Read the model definition and answer for the solid it produces. Units are mm, in the model's axes. A direction names the side the tool comes from. Give positions to 0.01 mm unless a question says otherwise; leave off trailing zeros. Loops run counter-clockwise (first coordinate to the right, second up) from the corner with the lowest first, then second, coordinate; pieces in that order, holes last. Notation, with made-up numbers: (75, 58.5) - (106, 58.5) arc R29 ccw to (106, 84.5) - close; hole circle Ø4 at (30.25, 24.5). An arc over 180 degrees is marked (long way). Write item = value, one per line.
```python
from build123d import *

# Parameters (mm, degrees)
SKETCH1_W           = 42
SKETCH1_H           = 40
SKETCH1_R           = 2
SKETCH1_R_2         = 4
BOSS_EXTRUDE1_DEPTH = 3
SKETCH2_W           = 3
SKETCH2_H           = 40
BOSS_EXTRUDE2_DEPTH = 38
SKETCH3_W           = 40
SKETCH3_H           = 3
BOSS_EXTRUDE3_DEPTH = 40
CUT_EXTRUDE3_DEPTH  = 3


with BuildPart() as part:
    # Sketch1 → Boss-Extrude1 (new body)
    with BuildSketch(Plane(origin=(0, 0, 0), x_dir=(1, 0, 0), z_dir=(0, 1, 0))):
        Rectangle(SKETCH1_W, SKETCH1_H)
        with Locations(Location((-16, 15, 0), (0, 0, 270))):
            Circle(SKETCH1_R, mode=Mode.SUBTRACT)
        with Locations(Location((-16, -15, 0), (0, 0, 270))):
            Circle(SKETCH1_R, mode=Mode.SUBTRACT)
        with Locations(Location((-11, 0, 0), (0, 0, 270))):
            Circle(SKETCH1_R_2, mode=Mode.SUBTRACT)
    extrude(amount=BOSS_EXTRUDE1_DEPTH)

    # Sketch2 → Boss-Extrude2 (add)
    with BuildSketch(Plane(origin=(0, 3, 0), x_dir=(1, 0, 0), z_dir=(0, 1, 0))):
        with Locations((19.5, 0)):
            Rectangle(SKETCH2_W, SKETCH2_H)
    extrude(amount=BOSS_EXTRUDE2_DEPTH)

    # Sketch3 → Boss-Extrude3 (add)
    with BuildSketch(Plane(origin=(21, 0, 0), x_dir=(0, 0, -1), z_dir=(1, 0, 0))):
        with Locations((0, 39.5)):
            Rectangle(SKETCH3_W, SKETCH3_H)
    extrude(amount=BOSS_EXTRUDE3_DEPTH)

    # Sketch8 → Cut-Extrude3 (cut)
    with BuildSketch(Plane.XZ.offset(-38)):
        Polygon((21, -20), (61, 20), (61, -20), align=None)
    extrude(amount=-CUT_EXTRUDE3_DEPTH, mode=Mode.SUBTRACT)


solid = part.part
```
1) The mould has two halves that part along Z. Classify faces 4 (the face through (-14, 1, -15)), 5 (the face through (20, 20, 20)), 6 (the face through (-2, 3, 0)): pulls with the +Z half, pulls with the -Z half, needs draft (parallel to the pull), parting line crosses it, or undercut.
Output:
face_4 = undercut
face_5 = pulls with the +Z half
face_6 = needs draft
2) Find the intervals of material crossed by probe 1 along X at (y, z) = (0.95, 15); probe 2 along X at (y, z) = (0.6, 0); probe 3 along X at (y, z) = (29.5, -5), in increasing order.
Output:
probe_1 = -21 to -18, -14 to 21
probe_2 = -21 to -15, -7 to 21
probe_3 = 18 to 21
3) A cutting plane is placed at D-D on x = 0. Determine the outline of the cut face in (y, z), then the cut area to 3 significant figures.
Output:
outline = (0, -20) - (3, -20) - (3, 20) - (0, 20) - close
area = 120 mm²
4) Each of these flat-tipped pins is pushed along its axis until it touches: P1, Ø10.5, axis at x = -11, z = 0, coming from the +Y side; P2, Ø2, axis at y = 6, z = -7, coming from the +X side; P3, Ø12, axis at x = 36.5, z = -6.5, coming from the -Y side. Where does it stop, or does it pass through?
Output:
P1 = 3
P2 = 21
P3 = 38
5) A cutting plane is placed at C-C on z = -8.5. Determine the outline of the cut face in (x, y).
Output:
outline = (-21, 0) - (21, 0) - (21, 38) - (32.5, 38) - (32.5, 41) - (18, 41) - (18, 3) - (-21, 3) - close
6) A tool of negligible diameter and unlimited length cuts with its end or side. For faces 1 (the face through (21, 19, 0)), 2 (the face through (-14.905, 1.479, -0.867)), 3 (the face through (18, 22, 0)), from which of +Z, -Z, +X, -X, +Y, -Y can it reach the whole face along a straight path? Write none if from no direction.
Output:
face_1 = +Z, -Z, +X, -Y
face_2 = +Y, -Y
face_3 = +Z, -Z, -X, +Y
7) A cutting plane is placed at A-A on z = 15. Determine the outline of the cut face in (x, y), then the cut area to 3 significant figures.
Output:
outline = (-21, 0) - (-18, 0) - (-18, 3) - (-21, 3) - close; (-14, 0) - (21, 0) - (21, 38) - (56, 38) - (56, 41) - (18, 41) - (18, 3) - (-14, 3) - close
area = 333 mm²
8) A cutting plane is placed at B-B on x = -11. Determine the outline of the cut face in (y, z), then the cut area to 3 significant figures.
Output:
outline = (0, -20) - (3, -20) - (3, -4) - (0, -4) - close; (0, 4) - (3, 4) - (3, 20) - (0, 20) - close
area = 96.0 mm²
